Input: part model. Units: mm. Frame: model coordinates. Face numbers are marked on the shaded views. A direction names the side the tool comes from. Round coordinates to 2 decimals unless told otherwise and drop trailing zeros. Loops run counter-clockwise (first coordinate to the right, second up) from the corner with the lowest first, then second, coordinate; pieces in that order, holes last. Notation, with made-up numbers: (15, -4) -> (59, -4) arc R18 cw to (59, 8) -> close; hole circle Ø10 at (8, -5.5). An arc over 180 degrees is marked (long way). Answer as a JSON object with one key per item and string values. Group by question number.
Item 1: Section query A-A on z = 19.5. Return loops of the section in (x, y) (3 decimals).
Item 2: Pin query (flat end, axial travel): pin 1 (3 mm diameter, centred on x = 47, z = 64.5, fed in from -Y) (3 decimals); pin 2 (10 mm diameter, centred on x = 66, y = 57.5, fed in from -Z). Return the tip coordinate at first contact, or that it passes through.
Item 3: Set-up query: the marked faces 1 and 2. Return all of +Z, -Z, +X, -X, +Y, -Y with unobstructed straight access to the full face (end or side cutting, diameter ignored); none if empty.
Item 4: Section query D-D on z = 70. Return loops of the section in (x, y) (3 decimals), and give its area (3 significant figures).
Item 5: Draft query along X for the marked faces 3, 4 and 5. Return one class per face: released by +X, released by -X, zero draft, split by the parting line, or undercut.
Item 6: Section query C-C on y = 48. Return loops of the section in (x, z) (3 decimals), and give its area (3 significant figures).
Item 7: Material intervals for line 1 (X direction, y = 71.5, z = 49.5) (3 decimals); line 2 (Y direction, x = 6, z = 60.5) (3 decimals), sorted ascending. Write a range as [from, to].
Item 8: Section query B-B on y = 70. Return loops of the section in (x, z) (3 decimals).
from build123d import *

# Parameters (mm, degrees)
F0_W     = 76.2
F0_H     = 76.2
F0_W_2   = 69.85
F0_H_2   = 69.85
F1_DEPTH = 76.2
F3_DEPTH = 25.4
F4_R     = 6.35
F5_DEPTH = 25.4
F4_R_2   = 14.351
F7_DEPTH = 25.4
F6_R     = 14.2875
F8_DEPTH = 25.4


with BuildPart() as f1:
    # F0 (on Top) → F1 (new body)
    with BuildSketch(Plane.XY):
        with Locations((38.1, 38.1)):
            Rectangle(F0_W, F0_H)
        with Locations((38.1, 38.1)):
            Rectangle(F0_W_2, F0_H_2, mode=Mode.SUBTRACT)
    extrude(amount=F1_DEPTH)

    # F2 (on face) → F3 (cut)
    with BuildSketch(Plane.XZ):
        Polygon((3.175, 76.2), (3.175, 14.417147), (3.175, 0), (73.025, 0), (73.025, 76.2), align=None)
    extrude(amount=-F3_DEPTH, mode=Mode.SUBTRACT)

    # F4 (on face) → F5 (cut)
    with BuildSketch(Plane.YZ.offset(3.175)):
        with Locations((66.675, 66.294)):
            Circle(F4_R)
        with Locations((66.427297, 9.525)):
            Circle(F4_R)
    extrude(amount=-F5_DEPTH, mode=Mode.SUBTRACT)

    # F4 (on face) → F7 (cut)
    with BuildSketch(Plane.YZ.offset(3.175)):
        with Locations((17.528682, 37.9095)):
            Circle(F4_R_2)
    extrude(amount=-F7_DEPTH, mode=Mode.SUBTRACT)

    # F6 (on face) → F8 (cut)
    with BuildSketch(Plane.YZ.offset(76.2)):
        with Locations((16.311424, 38.1)):
            Circle(F6_R)
    extrude(amount=-F8_DEPTH, mode=Mode.SUBTRACT)


solid = f1.part
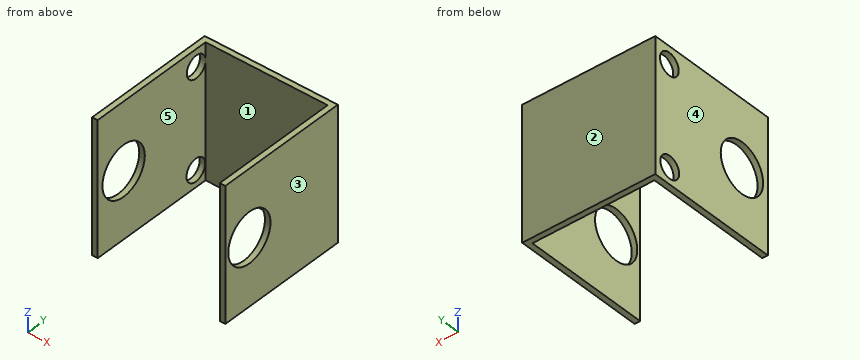
Solved:
{
 "1": {"outline": "(0, 0) -> (3.175, 0) -> (3.175, 73.025) -> (73.025, 73.025) -> (73.025, 0) -> (76.2, 0) -> (76.2, 76.2) -> (0, 76.2) -> close"},
 "2": {"pin 1": "y = 73.025", "pin 2": "through"},
 "3": {"face 1": "+Z, -Z, -Y", "face 2": "+Z, -Z, +X, -X, +Y"},
 "4": {"outline": "(0, 0) -> (3.175, 0) -> (3.175, 61.519) -> (0, 61.519) -> close; (0, 71.831) -> (3.175, 71.831) -> (3.175, 73.025) -> (73.025, 73.025) -> (73.025, 0) -> (76.2, 0) -> (76.2, 76.2) -> (0, 76.2) -> close", "area": "673 mm²"},
 "5": {"face 3": "released by +X", "face 4": "released by -X", "face 5": "undercut"},
 "6": {"outline": "(0, 0) -> (3.175, 0) -> (3.175, 76.2) -> (0, 76.2) -> close; (73.025, 0) -> (76.2, 0) -> (76.2, 76.2) -> (73.025, 76.2) -> close", "area": "484 mm²"},
 "7": {"line 1": "[0, 3.175], [73.025, 76.2]", "line 2": "[73.025, 76.2]"},
 "8": {"outline": "(0, 0) -> (3.175, 0) -> (3.175, 4.275) -> (0, 4.275) -> close; (0, 14.775) -> (3.175, 14.775) -> (3.175, 60.884) -> (0, 60.884) -> close; (0, 71.704) -> (3.175, 71.704) -> (3.175, 76.2) -> (0, 76.2) -> close; (73.025, 0) -> (76.2, 0) -> (76.2, 76.2) -> (73.025, 76.2) -> close"}
}
